The model under review builds one solid part; all positions refer to its coordinate system, in mm. A direction names the side the tool comes from. Round coordinates to 2 decimals unless told otherwise and drop trailing zeros. Loops run counter-clockwise (first coordinate to the right, second up) from the corner with the lowest first, then second, coordinate; pieces in that order, holes last. Notation, with made-up numbers: M -14.75,85 L 1.25,85 A6 ccw 1.25,90 Z; hole C 71.5,-20 d11. An arc over 180 degrees is marked long. Answer as a JSON object with one key per item and string values. Group by question number.
Item 1: To check wall thickness, follow line 1 (Y direction, x = -21.5, z = 23.25); line 2 (Y direction, x = -21, z = 7); line 3 (X direction, y = -97, z = 14). State the ranges of each line that lie inside material, in increasing order.
Item 2: Consider section C-C (z = 13.75). Give the boundary of the cut face in (x, y), and give its area (3 significant figures).
Item 3: The part is to be moulded in two halves that separate along X. For faces 3 (the face through (74.368, 114.847, 14.79)), 4 (the face through (-1, -5, 30)), 5 (the face through (-1, -120.193, 15)), say which applies: +X half, -X half, draft (parallel to the pull), parting line (faces both ways), or undercut.
Item 4: Tool access review of faces 1 (the face through (1, 120.856, 15)), 2 (the face through (-1, -60.193, 15)): name each direction out of +Z, -Z, +X, -X, +Y, -Y from which nothing blocks a thin tool from reaching the whole face with its end or side.
Item 5: Consider section B-B (x = -49.5). Give the boundary of the cut face in (y, z), and give its area (3 significant figures).
Item 6: Consider section A-A (y = -93). Give the boundary of the cut face in (x, z), and give its area (3 significant figures).
Item 7: Consider section D-D (x = 1.5). Give the boundary of the cut face in (y, z), and give its area (3 significant figures).
```python
from build123d import *

# Parameters (mm, degrees)
SKETCH_R     = 25
SKETCH_R_2   = 12
SKETCH_W     = 60
SKETCH_H     = 60
PAD_DEPTH    = 30
PAD001_DEPTH = 30


with BuildPart() as part:
    # Sketch → Pad (new body)
    with BuildSketch(Plane.XY):
        with BuildLine():
            Line((-59.342312, -134.143673), (59.515305, -134.143673))
            ThreePointArc((59.515305, -134.143673), (74.047401, -128.124281), (80.066793, -113.592185))
            Line((80.066793, -113.592185), (80.066793, 100.872214))
            ThreePointArc((80.066793, 100.872214), (74.213582, 115.003116), (60.08268, 120.856327))
            Line((60.08268, 120.856327), (-59.689381, 120.856327))
            ThreePointArc((-59.689381, 120.856327), (-74.003928, 114.927048), (-79.933207, 100.612501))
            Line((-79.933207, 100.612501), (-79.933207, -113.552778))
            ThreePointArc((-79.933207, -113.552778), (-73.902274, -128.112739), (-59.342312, -134.143673))
        make_face()
        with Locations((0.120778, 29.919195)):
            Circle(SKETCH_R, mode=Mode.SUBTRACT)
        with Locations((-53.325886, -24.171413)):
            Circle(SKETCH_R_2, mode=Mode.SUBTRACT)
        with Locations((55.271923, 86.295181)):
            Circle(SKETCH_R_2, mode=Mode.SUBTRACT)
        with Locations((-0.129082, -90.192567)):
            Rectangle(SKETCH_W, SKETCH_H, mode=Mode.SUBTRACT)
    extrude(amount=PAD_DEPTH)

    # Sketch → Pad001 (join)
    with BuildSketch(Plane.XY):
        with BuildLine():
            Line((-59.342312, -134.143673), (59.515305, -134.143673))
            ThreePointArc((59.515305, -134.143673), (74.047401, -128.124281), (80.066793, -113.592185))
            Line((80.066793, -113.592185), (80.066793, 100.872214))
            ThreePointArc((80.066793, 100.872214), (74.213582, 115.003116), (60.08268, 120.856327))
            Line((60.08268, 120.856327), (-59.689381, 120.856327))
            ThreePointArc((-59.689381, 120.856327), (-74.003928, 114.927048), (-79.933207, 100.612501))
            Line((-79.933207, 100.612501), (-79.933207, -113.552778))
            ThreePointArc((-79.933207, -113.552778), (-73.902274, -128.112739), (-59.342312, -134.143673))
        make_face()
        with Locations((0.120778, 29.919195)):
            Circle(SKETCH_R, mode=Mode.SUBTRACT)
        with Locations((-53.325886, -24.171413)):
            Circle(SKETCH_R_2, mode=Mode.SUBTRACT)
        with Locations((55.271923, 86.295181)):
            Circle(SKETCH_R_2, mode=Mode.SUBTRACT)
        with Locations((-0.129082, -90.192567)):
            Rectangle(SKETCH_W, SKETCH_H, mode=Mode.SUBTRACT)
    extrude(amount=PAD001_DEPTH)


solid = part.part
```
Geometry results:
{
 "1": {"line 1": "y = -134.14 to -120.19, -60.19 to 17.37, 42.47 to 120.86", "line 2": "y = -134.14 to -120.19, -60.19 to 16.54, 43.3 to 120.86", "line 3": "x = -79.93 to -30.13, 29.87 to 80.07"},
 "2": {"outline": "M -79.93,-113.55 A20.59 ccw -59.34,-134.14 L 59.52,-134.14 A20.55 ccw 80.07,-113.59 L 80.07,100.87 A19.98 ccw 60.08,120.86 L -59.69,120.86 A20.24 ccw -79.93,100.61 Z; hole C -53.33,-24.17 d24; hole M -30.13,-120.19 L 29.87,-120.19 L 29.87,-60.19 L -30.13,-60.19 Z; hole C 0.12,29.92 d50; hole C 55.27,86.3 d24", "area": "34,000 mm^2"},
 "3": {"face 3": "+X half", "face 4": "draft", "face 5": "undercut"},
 "4": {"face 1": "+Z, -Z, +X, -X, +Y", "face 2": "+Z, -Z"},
 "5": {"outline": "M -134.14,0 L -35.55,0 L -35.55,30 L -134.14,30 Z; M -12.8,0 L 120.86,0 L 120.86,30 L -12.8,30 Z", "area": "6,970 mm^2"},
 "6": {"outline": "M -79.93,0 L -30.13,0 L -30.13,30 L -79.93,30 Z; M 29.87,0 L 80.07,0 L 80.07,30 L 29.87,30 Z", "area": "3,000 mm^2"},
 "7": {"outline": "M -134.14,0 L -120.19,0 L -120.19,30 L -134.14,30 Z; M -60.19,0 L 4.96,0 L 4.96,30 L -60.19,30 Z; M 54.88,0 L 120.86,0 L 120.86,30 L 54.88,30 Z", "area": "4,350 mm^2"}
}
